```python
from build123d import *

# Parameters (mm, degrees)
F1_DEPTH      = 2
F2_DEPTH      = 4.2
F3_DEPTH      = 6.2
F4_DEPTH      = 6.2
F5_W          = 4
F5_H          = 2
F5_H_2        = 4
F6_DEPTH      = 2
F7_R          = 2.5
F7_R_2        = 1.5
F8_DEPTH      = 2.5
F9_DEPTH      = 4.5
F10_R         = 5
F12_START     = -1.7
F11_R         = 2.5
F11_R_2       = 1.5
F12_DEPTH     = 5.1
F13_DEPTH     = 4.2
F14_W         = 5.5
F14_H         = 2
F15_DEPTH     = 0.4
F16_T1_DEPTH  = 7.9494897428
F16_T3_DEPTH  = 7.9494897428
F17_S5_R      = 1.5
F17_T6_DEPTH  = 5
F17_S11_R     = 1.5
F17_T12_DEPTH = 5
F17_S17_R     = 1.5
F17_T18_DEPTH = 5


# Not quite as in the source:
# - a fillet or chamfer that OpenCascade refuses, or shapes differently, is made with other operations: its cross-section is extruded or revolved along the edge and cut away or added


with BuildPart() as f1:
    # F0 (on Top) → F1 (new body)
    with BuildSketch(Plane.XY):
        with BuildLine():
            Line((26, 14.25), (22.5, 14.25))
            ThreePointArc((22.5, 14.25), (23.9142135624, 13.6642135624), (24.5, 12.25))
            Line((24.5, 12.25), (24.5, -16.75))
            Line((24.5, -16.75), (30, -24.25))
            Line((30, -24.25), (30, 4.25))
            Line((30, 4.25), (26, 14.25))
        make_face()
    extrude(amount=F1_DEPTH)



with BuildPart() as f1b:
    # F0 (on Top) → F1, piece 2 (new body)
    with BuildSketch(Plane.XY):
        with BuildLine():
            Line((-22, 14.25), (-25.5, 14.25))
            Line((-25.5, 14.25), (-29.5, 4.25))
            Line((-29.5, 4.25), (-29.5, -24.25))
            Line((-29.5, -24.25), (-24, -16.75))
            Line((-24, -16.75), (-24, 12.25))
            ThreePointArc((-24, 12.25), (-23.4142135624, 13.6642135624), (-22, 14.25))
        make_face()
    extrude(amount=F1_DEPTH)


with BuildPart() as f1_1:
    add(f1.part)

    add(f1b.part)  # F2 merges F1b
    # F0 (on Top) → F2 (join)
    with BuildSketch(Plane.XY):
        Polygon((-29.5, 4.25), (-25.5, 14.25), (-22, 14.25), (22.5, 14.25), (26, 14.25), (30, 4.25), (30, -24.25), (30, -31.75), (34, -31.6827731092), (34, 5.0203296143), (27.1081318457, 28.25), (-24.2081318457, 28.25), (-33.5, 5.0203296143), (-33.5, -32.8172268908), (-29.5, -32.75), (-29.5, -24.25), align=None)
    extrude(amount=F2_DEPTH)

    # F3 (add): faces of the model
    f3_faces = [f1_1.faces().sort_by_distance(p)[0] for p in [
        (-33.5, -13.8984486382, 2.1),
        (-28.8540659229, 16.6351648071, 2.1),
    ]]
    extrude(f3_faces, amount=F3_DEPTH, dir=(-1, 0, 0))

    # F4 (add): faces of the model
    f4_faces = [f1_1.faces().sort_by_distance(p)[0] for p in [
        (34, -13.3312217475, 2.1),
        (30.5540659229, 16.6351648071, 2.1),
    ]]
    extrude(f4_faces, amount=F4_DEPTH, dir=(1, 0, 0))

    # F5 (on face) → F6 (join)
    with BuildSketch(Plane.XY.offset(4.2)):
        with Locations((-34.7, -26.75)):
            Rectangle(F5_W, F5_H)
        with Locations((35.2, -26.75)):
            Rectangle(F5_W, F5_H)
        with Locations((35.2, 4.25)):
            Rectangle(F5_W, F5_H_2)
        with Locations((-34.7, 4.25)):
            Rectangle(F5_W, F5_H_2)
    extrude(amount=F6_DEPTH)

    # F7 (on face) → F8 (cut)
    with BuildSketch(Plane(origin=(0, 0, 0), x_dir=(1, 0, 0), z_dir=(0, 0, -1))):
        with Locations((-34, 8.3172268908)):
            Circle(F7_R)
        with Locations((-34, 8.3172268908)):
            Circle(F7_R_2, mode=Mode.SUBTRACT)
        with Locations((34.5, 8.3172268908)):
            Circle(F7_R)
        with Locations((34.5, 8.3172268908)):
            Circle(F7_R_2, mode=Mode.SUBTRACT)
    extrude(amount=-F8_DEPTH, mode=Mode.SUBTRACT)

    # F9 (cut): faces of the model
    f9_faces = [f1_1.faces().sort_by_distance(p)[0] for p in [
        (-34, -8.3172268908, 0),
        (34.5, -8.3172268908, 0),
    ]]
    extrude(f9_faces, amount=-F9_DEPTH, mode=Mode.SUBTRACT)

    # F10
    f10_edges = [f1_1.edges().sort_by_distance(p)[0] for p in [
        (24.5, -16.75, 1),
        (-24, -16.75, 1),
    ]]
    fillet(f10_edges, radius=F10_R)

    # F11 (on face) → F12 (cut)
    with BuildSketch(Plane.XY.offset(4.2).offset(F12_START)):
        with Locations((0.25, 20.25)):
            Circle(F11_R)
        with Locations((0.25, 20.25)):
            Circle(F11_R_2, mode=Mode.SUBTRACT)
    extrude(amount=-F12_DEPTH, mode=Mode.SUBTRACT)

    # F11 (on face) → F13 (cut)
    with BuildSketch(Plane.XY.offset(4.2)):
        with Locations((0.25, 20.25)):
            Circle(F11_R_2)
    extrude(amount=-F13_DEPTH, mode=Mode.SUBTRACT)

    # F14 (on face) → F15 (join)
    with BuildSketch(Plane.XY.offset(2)):
        with Locations((27.25, -5.25)):
            Rectangle(F14_W, F14_H)
        with Locations((-26.75, -5.25)):
            Rectangle(F14_W, F14_H)
    extrude(amount=F15_DEPTH)

    # F16: fillet of radius 1.4 on 4 edges, made by hand

    # F16_s2 → F16_t1 (cut)
    with BuildSketch(Plane.YZ.offset(-29.5)):
        with BuildLine():
            ThreePointArc((-6.25, 2), (-5.7993543651, 2.2961481397), (-5.2702041029, 2.4))
            Line((-5.2702041029, 2.4), (-6.25, 2.4))
            Line((-6.25, 2.4), (-6.25, 2))
        make_face()
        with BuildLine():
            ThreePointArc((-5.2297958971, 2.4), (-4.7006456349, 2.2961481397), (-4.25, 2))
            Line((-4.25, 2), (-4.25, 2.4))
            Line((-4.25, 2.4), (-5.2297958971, 2.4))
        make_face()
    extrude(amount=F16_T1_DEPTH, mode=Mode.SUBTRACT)

    # F16_s4 → F16_t3 (cut)
    with BuildSketch(Plane.YZ.offset(22.0505102572)):
        with BuildLine():
            ThreePointArc((-4.25, 2), (-4.7006456349, 2.2961481397), (-5.2297958971, 2.4))
            Line((-5.2297958971, 2.4), (-4.25, 2.4))
            Line((-4.25, 2.4), (-4.25, 2))
        make_face()
        with BuildLine():
            ThreePointArc((-5.2702041029, 2.4), (-5.7993543651, 2.2961481397), (-6.25, 2))
            Line((-6.25, 2), (-6.25, 2.4))
            Line((-6.25, 2.4), (-5.2702041029, 2.4))
        make_face()
    extrude(amount=F16_T3_DEPTH, mode=Mode.SUBTRACT)

    # F17: chamfer of 1.2 on 3 edges, made by hand


with BuildPart() as f17_tool2:
    # F17_s3 → F17_t4 (revolve)
    with BuildSketch(Plane.XZ.offset(8.3172268908)):
        Polygon((-31.5, 1.3), (-32.7, 2.5), (-31.5, 2.5), align=None)
    revolve(axis=Axis((-34, -8.3172268908, 2.5), (0, 0, -1)))

    # F17_s5 → F17_t6 (cut, symmetric)
    with BuildSketch(Plane.XY.offset(1.9)):
        with Locations((-34, -8.3172268908)):
            Circle(F17_S5_R)
    extrude(amount=F17_T6_DEPTH, both=True, mode=Mode.SUBTRACT)


with BuildPart() as f1_2:
    add(f1_1.part)

    # F17_t1: union F17_tool2
    add(f17_tool2.part)


with BuildPart() as f17_tool8:
    # F17_s9 → F17_t10 (revolve)
    with BuildSketch(Plane.XZ.offset(8.3172268908)):
        Polygon((37, 1.3), (35.8, 2.5), (37, 2.5), align=None)
    revolve(axis=Axis((34.5, -8.3172268908, 2.5), (0, 0, -1)))

    # F17_s11 → F17_t12 (cut, symmetric)
    with BuildSketch(Plane.XY.offset(1.9)):
        with Locations((34.5, -8.3172268908)):
            Circle(F17_S11_R)
    extrude(amount=F17_T12_DEPTH, both=True, mode=Mode.SUBTRACT)


with BuildPart() as f1_3:
    add(f1_2.part)

    # F17_t7: union F17_tool8
    add(f17_tool8.part)


with BuildPart() as f17_tool14:
    # F17_s15 → F17_t16 (revolve)
    with BuildSketch(Plane.XZ.offset(-20.25)):
        Polygon((2.75, 1.3), (1.55, 2.5), (2.75, 2.5), align=None)
    revolve(axis=Axis((0.25, 20.25, 2.5), (0, 0, 1)))

    # F17_s17 → F17_t18 (cut, symmetric)
    with BuildSketch(Plane.XY.offset(1.9)):
        with Locations((0.25, 20.25)):
            Circle(F17_S17_R)
    extrude(amount=F17_T18_DEPTH, both=True, mode=Mode.SUBTRACT)


with BuildPart() as f1_4:
    add(f1_3.part)

    # F17_t13: union F17_tool14
    add(f17_tool14.part)


solid = f1_4.part
```
Verification items for the finished model (mm, model axes). A direction names the side the tool comes from. Round coordinates to 2 decimals unless told otherwise and drop trailing zeros. Order: outer loops, then holes, each group sorted by start corner. A loop starts at its lowest first (then second) coordinate and runs counter-clockwise, first axis right, second up. Notation, with made-up numbers: (29.5, -25.5) - (85.5, -25.5) arc R35 ccw to (85.5, 6.5) - close; hole circle Ø11 at (22, 49). An arc over 180 degrees is marked (long way). Use CSV: the item, a comma, the result in double quotes.
(1) Mould release check, pull along Y, two halves, no side actions. Record for faces 1 (the face through (35, -27.75, 5)), 2 (the face through (33.31, -9.23, 3.26)), 3 (the face through (40.2, -14, 2)): released by +Y, released by -Y, zero draft, split by the parting line, or undercut.
Entries:
face 1,"released by -Y"
face 2,"undercut"
face 3,"zero draft"
(2) Gauge pin test, flat ends, axial feed: pin 1 Ø1 at (y, z) = (5, 5) entering from -X; pin 2 Ø5 at (x, y) = (24.5, -19.5) entering from +Z; pin 3 Ø1.6 at (x, z) = (-34, 5.5) entering from -Y. Record the tip position at first contact, or that the pin passes through.
Entries:
pin 1,"x = -36.7"
pin 2,"z = 2"
pin 3,"y = -27.75"
(3) Section check B-B on y = 9. Record the boundary of the cut face in (x, z), and give its area (3 significant figures).
Entries:
outline,"(-38.11, 0) - (-24, 0) - (-24, 2) - (-27.6, 2) - (-27.6, 4.2) - (-38.11, 4.2) - close; (24.5, 0) - (39.02, 0) - (39.02, 4.2) - (28.1, 4.2) - (28.1, 2) - (24.5, 2) - close"
area,"104 mm^2"
(4) Thickness scan on probe 1 along X at (y, z) = (2.5, 1.5); probe 2 along X at (y, z) = (-8, 1); probe 3 along X at (y, z) = (-24.5, 2.25). Record the ranges inside material, lowest first. Write a range as from..to.
Entries:
probe 1,"-39.7..-24, 24.5..40.2"
probe 2,"-39.7..-36.48, -31.52..-24, 24.5..32.02, 36.98..40.2"
probe 3,"-39.7..-29.5, 30..40.2"
(5) Section check C-C on x = 11. Record the boundary of the cut face in (y, z), and give its area (3 significant figures).
Entries:
outline,"(14.25, 0) - (28.25, 0) - (28.25, 4.2) - (14.25, 4.2) - close"
area,"58.8 mm^2"
(6) Access from +Z, -Z, +X, -X, +Y, -Y to the whole of each face (thin tool, end or side, straight path). Record for faces 4 (the face through (-24, -2, 1)), 5 (the face through (35, 6.25, 5)), 6 (the face through (27, 3, 2)), 7 (the face through (-36.7, -27, 5)).
Entries:
face 4,"+Z, -Z, -Y"
face 5,"+Z, +X, -X, +Y"
face 6,"+Z"
face 7,"+Z, -X, +Y, -Y"
(7) Section check A-A on x = 0.25. Record the boundary of the cut face in (y, z).
Entries:
outline,"(14.25, 0) - (17.75, 0) - (17.75, 1.3) - (18.75, 2.3) - (18.75, 4.2) - (14.25, 4.2) - close; (21.75, 2.3) - (22.75, 1.3) - (22.75, 0) - (28.25, 0) - (28.25, 4.2) - (21.75, 4.2) - close"
